Part model, mm, in its own coordinate system. A direction names the side the tool comes from. Round coordinates to 2 decimals unless told otherwise and drop trailing zeros. Order: outer loops, then holes, each group sorted by start corner. A loop starts at its lowest first (then second) coordinate and runs counter-clockwise, first axis right, second up. Notation, with made-up numbers: M 67,3.5 L 88,3.5 A31 ccw 88,31.5 Z; hole C 69.25,-16.75 d8. An arc over 180 degrees is marked long. Write each question's results on one line, items separated by ' | '. Start each with the question number.
1. Which spindle directions (+Z, -Z, +X, -X, +Y, -Y) get a long thin tool onto all of the face, cutting with end or side? Do faces 1 (the face through (-13.38, -25.73, -55.99)), 2 (the face through (-8.071, 61.472, -7.395)). Say none if no direction does.
2. Drop flat-ended pins along their axis: pin 1 Ø2 at (y, z) = (18.5, -18) entering from +X; pin 2 Ø3 at (x, z) = (44, -23) entering from -Y; pin 3 Ø8 at (x, z) = (38, -13) entering from +Y. Give the stop position or say it passes through.
3. Band-saw the part on D-D, the plane x = -31.5. List the corners of the cut face in (y, z), then the cut area to 3 significant figures.
4. Probe L1, parallel to Z at x = -9, y = -55; L2, parallel to Y at x = 0, z = -19.5; L3, parallel to X at y = 2, z = -4.5. List the from-to ranges inside material, lowest first. Write a range as [from, to].
5. Two-plate mould, pull along Z, no slides. Class faces 3 (the face through (-9.83, -44.27, 0.99)), 4 (the face through (-28, -13, -57)), 5 (the face through (4, -46, 0)): +Z half, -Z half, draft (parallel to the pull), parting line (faces both ways), or undercut.
6. Band-saw the part on A-A, the plane x = 0. List the corners of the cut face in (y, z), then the cut area to 3 significant figures.
7. Band-saw the part on C-C, the plane z = -49.5. List the corners of the cut face in (x, y).
```python
from build123d import *

# Parameters (mm, degrees)
SKETCH1_R           = 64
SKETCH1_R_2         = 62
BOSS_EXTRUDE1_DEPTH = 55
SKETCH2_R           = 62
SKETCH2_R_2         = 60
BOSS_EXTRUDE2_DEPTH = 10
SKETCH3_R           = 64
SKETCH3_R_2         = 45.35
BOSS_EXTRUDE3_DEPTH = 2
SKETCH4_R           = 64
SKETCH4_R_2         = 29
BOSS_EXTRUDE4_DEPTH = 2


with BuildPart() as part:
    # Sketch1 → Boss-Extrude1 (new body)
    with BuildSketch(Plane.XY):
        Circle(SKETCH1_R)
        Circle(SKETCH1_R_2, mode=Mode.SUBTRACT)
    extrude(amount=-BOSS_EXTRUDE1_DEPTH)

    # Sketch2 → Boss-Extrude2 (add)
    with BuildSketch(Plane(origin=(0, 0, -15), x_dir=(-1, 0, 0), z_dir=(0, 0, -1))):
        Circle(SKETCH2_R)
        Circle(SKETCH2_R_2, mode=Mode.SUBTRACT)
    extrude(amount=BOSS_EXTRUDE2_DEPTH)

    # Sketch3 → Boss-Extrude3 (add)
    with BuildSketch(Plane.XY):
        Circle(SKETCH3_R)
        Circle(SKETCH3_R_2, mode=Mode.SUBTRACT)
    extrude(amount=BOSS_EXTRUDE3_DEPTH)

    # Sketch4 → Boss-Extrude4 (add)
    with BuildSketch(Plane(origin=(0, 0, -55), x_dir=(-1, 0, 0), z_dir=(0, 0, -1))):
        Circle(SKETCH4_R)
        Circle(SKETCH4_R_2, mode=Mode.SUBTRACT)
    extrude(amount=BOSS_EXTRUDE4_DEPTH)


solid = part.part
```
Solution:
1) face 1: +Z, -Z | face 2: none
2) pin 1: x = 61.56 | pin 2: y = -47.85 | pin 3: y = 54.22
3) outline: M -55.71,-57 L 55.71,-57 L 55.71,2 L 32.62,2 L 32.62,0 L 53.4,0 L 53.4,-15 L 51.07,-15 L 51.07,-25 L 53.4,-25 L 53.4,-55 L -53.4,-55 L -53.4,-25 L -51.07,-25 L -51.07,-15 L -53.4,-15 L -53.4,0 L -32.62,0 L -32.62,2 L -55.71,2 Z | area: 616 mm^2
4) L1: [-57, -55], [0, 2] | L2: [-64, -60], [60, 64] | L3: [-63.97, -61.97], [61.97, 63.97]
5) face 3: draft | face 4: -Z half | face 5: undercut
6) outline: M -64,-57 L -29,-57 L -29,-55 L -62,-55 L -62,-25 L -60,-25 L -60,-15 L -62,-15 L -62,0 L -45.35,0 L -45.35,2 L -64,2 Z; M 29,-57 L 64,-57 L 64,2 L 45.35,2 L 45.35,0 L 62,0 L 62,-15 L 60,-15 L 60,-25 L 62,-25 L 62,-55 L 29,-55 Z | area: 475 mm^2
7) outline: C 0,0 d128; hole C 0,0 d124
